```python
from build123d import *

# Parameters (mm, degrees)
SKETCH3_R             = 2.6
BOSS_EXTRUDE1_DEPTH   = 6
FILLET1_R             = 10
M3_CLEARANCE_HOLE1_D  = 3.2
M4X0_7_TAPPED_HOLE1_D = 3.3
FILLET2_R             = 2
SKETCH5_R             = 5
COUNTERBORE_DEPTH     = 1.5


with BuildPart() as part:
    # Sketch3 → Boss-Extrude1 (new body)
    with BuildSketch(Plane(origin=(0, 0, 0), x_dir=(1, 0, 0), z_dir=(0, 1, 0))):
        Polygon((0, 0), (78.5, 0), (78.5, 70), (0, 70), (-13.5, 70), (-13.5, 25), (0, 25), align=None)
        with Locations((10, 56)):
            Circle(SKETCH3_R, mode=Mode.SUBTRACT)
        with Locations((10, 10)):
            Circle(SKETCH3_R, mode=Mode.SUBTRACT)
        with Locations((68.5, 10)):
            Circle(SKETCH3_R, mode=Mode.SUBTRACT)
        with Locations((30, 10)):
            Circle(SKETCH3_R, mode=Mode.SUBTRACT)
        with BuildLine():
            Line((47.5, 59.5), (57.5, 59.5))
            ThreePointArc((57.5, 59.5), (69.5, 47.5), (57.5, 35.5))
            Line((57.5, 35.5), (47.5, 35.5))
            ThreePointArc((47.5, 35.5), (35.5, 47.5), (47.5, 59.5))
        make_face(mode=Mode.SUBTRACT)
        with BuildLine():
            Line((32, 64.6), (42, 64.6))
            ThreePointArc((42, 64.6), (43.6, 63), (42, 61.4))
            Line((42, 61.4), (32, 61.4))
            ThreePointArc((32, 61.4), (30.4, 63), (32, 64.6))
        make_face(mode=Mode.SUBTRACT)
        with BuildLine():
            Line((63, 64.6), (73, 64.6))
            ThreePointArc((73, 64.6), (74.6, 63), (73, 61.4))
            Line((73, 61.4), (63, 61.4))
            ThreePointArc((63, 61.4), (61.4, 63), (63, 64.6))
        make_face(mode=Mode.SUBTRACT)
        with BuildLine():
            Line((63, 33.6), (73, 33.6))
            ThreePointArc((73, 33.6), (74.6, 32), (73, 30.4))
            Line((73, 30.4), (63, 30.4))
            ThreePointArc((63, 30.4), (61.4, 32), (63, 33.6))
        make_face(mode=Mode.SUBTRACT)
        with BuildLine():
            Line((32, 33.6), (42, 33.6))
            ThreePointArc((42, 33.6), (43.6, 32), (42, 30.4))
            Line((42, 30.4), (32, 30.4))
            ThreePointArc((32, 30.4), (30.4, 32), (32, 33.6))
        make_face(mode=Mode.SUBTRACT)
    extrude(amount=BOSS_EXTRUDE1_DEPTH)

    # Fillet1
    fillet1_edges = [part.edges().sort_by_distance(p)[0] for p in [
        (0, 3, -25),
    ]]
    fillet(fillet1_edges, radius=FILLET1_R)

    # M3 Clearance Hole1 (through all)
    with Locations(Plane(origin=(0, 6, 0), x_dir=(1, 0, 0), z_dir=(0, 1, 0))):
        with Locations((10, 64.325), (-6.5, 64.325)):
            Hole(M3_CLEARANCE_HOLE1_D / 2)

    # M4x0.7 Tapped Hole1 (through all)
    with Locations(Plane(origin=(0, 6, 0), x_dir=(1, 0, 0), z_dir=(0, 1, 0))):
        with Locations((-6.5, 46.325), (10, 35.7)):
            Hole(M4X0_7_TAPPED_HOLE1_D / 2)

    # Fillet2
    fillet2_edges = [part.edges().sort_by_distance(p)[0] for p in [
        (-13.5, 3, -25),
        (-13.5, 3, -70),
        (78.5, 3, -70),
        (78.5, 3, 0),
        (0, 3, 0),
    ]]
    fillet(fillet2_edges, radius=FILLET2_R)

    # Sketch5 → Counterbore (cut)
    with BuildSketch(Plane(origin=(0, 6, 0), x_dir=(1, 0, 0), z_dir=(0, 1, 0))):
        with Locations((10, 56)):
            Circle(SKETCH5_R)
        with Locations((10, 10)):
            Circle(SKETCH5_R)
        with Locations((30, 10)):
            Circle(SKETCH5_R)
        with Locations((68.5, 10)):
            Circle(SKETCH5_R)
    extrude(amount=-COUNTERBORE_DEPTH, mode=Mode.SUBTRACT)


solid = part.part
```
Verification items for the finished model (mm, model axes). A direction names the side the tool comes from. Round coordinates to 2 decimals unless told otherwise and drop trailing zeros. Write each loop counter-clockwise with the first axis right and the second up, starting at its lowest first coordinate (ties: lowest second). Pieces come first, ordered by that corner, then holes. Notation, with made-up numbers: (-8, 14.25) -> (2, 14.25) arc R18 cw to (2, 29.25) -> close; hole circle Ø2 at (67, 31). An arc over 180 degrees is marked (long way). Write each question's results on one line, items separated by ' | '.
Q1. Go/stop test with flat-tipped pins: pin 1 Ø5 at (x, z) = (11, -12) entering from +Y; pin 2 Ø1 at (y, z) = (3, -20.5) entering from -X. Record where each tip stops, or that it passes through.
Derived:
pin 1: stops at y = 4.5 | pin 2: stops at x = -2
Q2. Access from +Z, -Z, +X, -X, +Y, -Y to the whole of each face (thin tool, end or side, straight path). Record for faces 5 (the face through (32, 6, -35)), 6 (the face through (14.77, 5.26, -11.5)), 7 (the face through (53, 3, -35.5)).
Derived:
face 5: +Z, -Z, +X, -X, +Y | face 6: +Y | face 7: +Y, -Y
Q3. Sectioned sample at C-C, the plane z = -43. Record the boundary of the cut face in (x, y).
Derived:
outline: (-13.5, 0) -> (36.38, 0) -> (36.38, 6) -> (-13.5, 6) -> close; (68.62, 0) -> (78.5, 0) -> (78.5, 6) -> (68.62, 6) -> close
Q4. Draft check along Z on faces 1 (the face through (0, 3, -9)), 2 (the face through (25, 5, -10)), 3 (the face through (-12.9, 3.04, -25.57)), 4 (the face through (61.4, 3, -63)). Enter one of: released by +Z, released by -Z, zero draft, split by the parting line, or undercut.
Derived:
face 1: zero draft | face 2: undercut | face 3: released by +Z | face 4: undercut
Q5. Sectioned sample at A-A, the plane x = 10. Record the boundary of the cut face in (y, z) (3 decimals), and give its area (3 significant figures).
Derived:
outline: (0, -70) -> (6, -70) -> (6, -65.925) -> (0, -65.925) -> close; (0, -62.725) -> (6, -62.725) -> (6, -61) -> (4.5, -61) -> (4.5, -58.6) -> (0, -58.6) -> close; (0, -53.4) -> (4.5, -53.4) -> (4.5, -51) -> (6, -51) -> (6, -37.35) -> (0, -37.35) -> close; (0, -34.05) -> (6, -34.05) -> (6, -15) -> (4.5, -15) -> (4.5, -12.6) -> (0, -12.6) -> close; (0, -7.4) -> (4.5, -7.4) -> (4.5, -5) -> (6, -5) -> (6, 0) -> (0, 0) -> close | area: 304 mm²
Q6. Thickness scan on probe 1 along Z at (x, y) = (34.5, 4.4); probe 2 along Z at (x, y) = (10, 5.55) (3 decimals); probe 3 along X at (y, z) = (2.55, -10). Record the ranges inside material, lowest first.
Derived:
probe 1: z = -70 to -64.6, -61.4 to -33.6, -30.4 to 0 | probe 2: z = -70 to -65.925, -62.725 to -61, -51 to -37.35, -34.05 to -15, -5 to 0 | probe 3: x = 0 to 7.4, 12.6 to 27.4, 32.6 to 65.9, 71.1 to 78.5
Q7. Sectioned sample at D-D, the plane x = -6.5. Record the boundary of the cut face in (y, z) (1 decimal), and give its area (3 significant figures).
Derived:
outline: (0, -70) -> (6, -70) -> (6, -65.9) -> (0, -65.9) -> close; (0, -62.7) -> (6, -62.7) -> (6, -48) -> (0, -48) -> close; (0, -44.7) -> (6, -44.7) -> (6, -24.4) -> (0, -24.4) -> close | area: 235 mm²
Q8. Sectioned sample at B-B, the plane z = -10. Record the boundary of the cut face in (x, y).
Derived:
outline: (0, 0) -> (7.4, 0) -> (7.4, 4.5) -> (5, 4.5) -> (5, 6) -> (0, 6) -> close; (12.6, 0) -> (27.4, 0) -> (27.4, 4.5) -> (25, 4.5) -> (25, 6) -> (15, 6) -> (15, 4.5) -> (12.6, 4.5) -> close; (32.6, 0) -> (65.9, 0) -> (65.9, 4.5) -> (63.5, 4.5) -> (63.5, 6) -> (35, 6) -> (35, 4.5) -> (32.6, 4.5) -> close; (71.1, 0) -> (78.5, 0) -> (78.5, 6) -> (73.5, 6) -> (73.5, 4.5) -> (71.1, 4.5) -> close
